from build123d import *

# Parameters (mm, degrees)
CUT_EXTRUDE1_START = -2.5
CUT_EXTRUDE1_DEPTH = 2.5
SKETCH4_R          = 2.309401077
CUT_EXTRUDE2_DEPTH = 0.5
CUT_EXTRUDE2_TAPER = 45


with BuildPart() as part:
    # Sketch2 → Revolve1 (revolve)
    with BuildSketch(Plane(origin=(0, 0, 0), x_dir=(0, 0, -1), z_dir=(1, 0, 0))):
        Polygon((-9.75, 4.25), (-5.25, 4.25), (-5, 4), (-5, 2.5), (9.2, 2.5), (10, 1.7), (10, 0), (-10, 0), (-10, 4), align=None)
    revolve(axis=Axis((0, 0, -10), (0, 0, 1)))

    # Sketch3 → Cut-Extrude1 (cut)
    with BuildSketch(Plane.XY.offset(10).offset(CUT_EXTRUDE1_START)):
        Polygon((0, 2.309401077), (-2, 1.154700538), (-2, -1.154700538), (0, -2.309401077), (2, -1.154700538), (2, 1.154700538), align=None)
    extrude(amount=CUT_EXTRUDE1_DEPTH, mode=Mode.SUBTRACT)

    # Sketch4 → Cut-Extrude2 (cut)
    with BuildSketch(Plane.XY.offset(10)):
        Circle(SKETCH4_R)
    extrude(amount=-CUT_EXTRUDE2_DEPTH, taper=CUT_EXTRUDE2_TAPER, mode=Mode.SUBTRACT)


solid = part.part
Work out the finished part from the listing and answer in its coordinate system (mm). A direction names the side the tool comes from. Round coordinates to 2 decimals unless told otherwise and drop trailing zeros. Loops run counter-clockwise (first coordinate to the right, second up) from the corner with the lowest first, then second, coordinate; pieces in that order, holes last. Notation, with made-up numbers: (10, 7) -> (15, 7) arc R22 ccw to (15, 21) -> close; hole circle Ø9 at (52, -4.75). An arc over 180 degrees is marked (long way). Use one line per item in the form item = value.
(1) Flat-ended cylindrical pins translate along their axes: P1, Ø2, axis at x = 0, y = 0.5, coming from the +Z side; P2, Ø1.5, axis at x = 2, y = 2.5, coming from the -Z side; P3, Ø1.5, axis at x = 0, y = 2, coming from the +Z side; P4, Ø1.5, axis at x = 0.5, y = -3, coming from the -Z side. Find the tip coordinate at first contact, or state that the pin passes through.
Answer list:
P1 = 7.5
P2 = -9.25
P3 = 10
P4 = -9.41
(2) Find section A-A on y = 0. Give the vertices of the cut face in (x, z).
Answer list:
outline = (-4.25, 5.25) -> (-4, 5) -> (-2.5, 5) -> (-2.5, -9.2) -> (-1.7, -10) -> (1.7, -10) -> (2.5, -9.2) -> (2.5, 5) -> (4, 5) -> (4.25, 5.25) -> (4.25, 9.75) -> (4, 10) -> (2.31, 10) -> (2, 9.69) -> (2, 7.5) -> (-2, 7.5) -> (-2, 9.69) -> (-2.31, 10) -> (-4, 10) -> (-4.25, 9.75) -> close
(3) Straight lines are drawn through the part: line 1 (Z direction, x = 3, y = -1.5); line 2 (X direction, y = 0, z = 2); line 3 (Z direction, x = 0.5, y = -0.5). For each, find the intervals that lie inside material, in ascending order.
Answer list:
line_1 = 5 to 10
line_2 = -2.5 to 2.5
line_3 = -10 to 7.5
(4) A tool of negligible diameter and unlimited length cuts with its end or side. For faces 1 (the cylindrical face through (-3.584, 2.285, 7.469)), 2 (the flat face through (-2, 2, 5)), 3 (the flat face through (2, 0, 9)), from which of +Z, -Z, +X, -X, +Y, -Y can it reach the whole face along a straight path? Write none if from no direction.
Answer list:
face_1 = +Z, -Z
face_2 = -Z
face_3 = +Z
(5) For a pull along X with two mould halves and no side action, classify faces 4 (the flat face through (0, 0, -10)), 5 (the flat face through (0, 0, 7.5)), 6 (the cylindrical face through (2.44, -0.54, -2.2)) as released by +X, released by -X, zero draft, split by the parting line, or undercut.
Answer list:
face_4 = zero draft
face_5 = undercut
face_6 = split by the parting line
(6) Find section B-B on z = -7.5. Give the vertices of the cut face in (x, y), then the cut area to 3 significant figures.
Answer list:
outline = circle Ø5 at (0, 0)
area = 19.6 mm2
